Geometry check sheet. Reference: the model listing, model coordinates, mm. A direction names the side the tool comes from. Coordinates: 2 decimals unless noted, no trailing zeros. Put each result on its own line as item: value. Start each with the question number.
1) Mould release check, pull along Y, two halves, no side actions. Record for faces 1 (the cylindrical face through (6.1, 1210.4, -8)), 2 (the flat face through (0, 1223.962, 0)), 3 (the flat face through (0, 0, 0)): released by +Y, released by -Y, zero draft, split by the parting line, or undercut.
2) Scan lines: line 1 along Y through (x, z) = (0, -6); line 2 along Z through (x, y) = (-13, 240); line 3 along X through (y, z) = (261.5, 11). Record each from-to range of solid material in increasing order.
3) Set-up check for faces 4 (the cylindrical face through (6.11, 13.57, -8)), 5 (the cylindrical face through (6.11, 13.57, 8)): record each of +Z, -Z, +X, -X, +Y, -Y from which the full face is reachable in a straight line by a thin tool's end or side.
4) Gauge pin test, flat ends, axial feed: pin 1 (12 mm diameter, centred on x = 0, z = 8.5, fed in from +Y); pin 2 (3 mm diameter, centred on y = 825, z = 1, fed in from +X); pin 3 (4 mm diameter, centred on x = -1, y = 323.5, fed in from +Z); pin 4 (11 mm diameter, centred on x = -2, y = 1200, fed in from -Z). Record the tip position at first contact, or that the pin passes through.
from build123d import *

# Parameters (mm, degrees)
BOSS_EXTRUDE1_DEPTH     = 1223.9625
SKETCH3_R               = 10.287
CUT_EXTRUDE1_DEPTH      = 16.51
MIRROR2_COPY_1_SKETCH_R = 10.287
MIRROR2_COPY_1_DEPTH    = 16.51


with BuildPart() as part:
    # Sketch2 → Boss-Extrude1 (new body)
    with BuildSketch(Plane(origin=(0.594697292, 0, 0.594697292), x_dir=(1, 0, 0), z_dir=(0, 1, 0))):
        Polygon((-19.644697292, 19.644697292), (-4.658697292, 19.644697292), (-4.658697292, 15.580697292), (-12.707015333, 15.580697292), (-4.477415333, 7.351097292), (3.288020749, 7.351097292), (11.517620749, 15.580697292), (3.469302708, 15.580697292), (3.469302708, 19.644697292), (18.455302708, 19.644697292), (18.455302708, 4.658697292), (14.391302708, 4.658697292), (14.391302708, 12.707015333), (6.161702708, 4.477415333), (6.161702708, -3.288020749), (14.391302708, -11.517620749), (14.391302708, -3.469302708), (18.455302708, -3.469302708), (18.455302708, -18.455302708), (3.469302708, -18.455302708), (3.469302708, -14.391302708), (11.517620749, -14.391302708), (3.288020749, -6.161702708), (-4.477415333, -6.161702708), (-12.707015333, -14.391302708), (-4.658697292, -14.391302708), (-4.658697292, -18.455302708), (-19.644697292, -18.455302708), (-19.644697292, -3.469302708), (-15.580697292, -3.469302708), (-15.580697292, -11.517620749), (-7.351097292, -3.288020749), (-7.351097292, 4.477415333), (-15.580697292, 12.707015333), (-15.580697292, 4.658697292), (-19.644697292, 4.658697292), align=None)
    extrude(amount=BOSS_EXTRUDE1_DEPTH)

    # Sketch3 → Cut-Extrude1 (cut)
    with BuildSketch(Plane.XY.offset(19.05)):
        with Locations(Location((0, 21.844, 0), (0, 0, 48.944473627))):
            Circle(SKETCH3_R)
    cut_extrude1 = extrude(amount=-CUT_EXTRUDE1_DEPTH, mode=Mode.SUBTRACT)

    # Mirror1: Cut-Extrude1 across plane
    add(cut_extrude1.mirror(Plane.XY), mode=Mode.SUBTRACT)

    # Mirror2: Cut-Extrude1 across plane
    add(cut_extrude1.mirror(Plane.ZX.offset(611.98125)), mode=Mode.SUBTRACT)

    # Mirror2 copy 1 sketch → Mirror2 copy 1 (cut)
    with BuildSketch(Plane(origin=(0, 1223.9625, -19.05), x_dir=(1, 0, 0), z_dir=(0, 0, -1))):
        with Locations(Location((0, 21.844, 0), (0, 0, 48.944473627))):
            Circle(MIRROR2_COPY_1_SKETCH_R)
    extrude(amount=-MIRROR2_COPY_1_DEPTH, mode=Mode.SUBTRACT)


solid = part.part
Answer key:
1. face 1: undercut
1. face 2: released by +Y
1. face 3: released by -Y
2. line 1: y = 0 to 11.56, 32.13 to 1191.83, 1212.41 to 1223.96
2. line 2: z = -19.05 to -10.13, 10.13 to 19.05
2. line 3: x = -19.05 to -14.99, -13.87 to -8.13, 8.13 to 13.87, 14.99 to 19.05
3. face 4: -Z
3. face 5: +Z
4. pin 1: stops at y = 1223.96
4. pin 2: stops at x = 6.76
4. pin 3: stops at z = 6.76
4. pin 4: stops at z = -2.54
